Check sheet for the modelled part. Datum: model origin and axes. Units: mm. A direction names the side the tool comes from. Coordinates: 2 decimals unless noted, no trailing zeros. Loops run counter-clockwise (first coordinate to the right, second up) from the corner with the lowest first, then second, coordinate; pieces in that order, holes last. Notation, with made-up numbers: M 7.5,58.5 L 16.5,58.5 A18 ccw 16.5,65.5 Z; hole C 33.5,24 d7. An arc over 180 degrees is marked long. Return JSON: item names as keys, results as strings.
from build123d import *

# Parameters (mm, degrees)
BASE_FLANGE1_DEPTH   = 10
EDGE_FLANGE1_START   = -322.556390977
EDGE_FLANGE1_DEPTH   = 500
EDGE_FLANGE1_2_DEPTH = 500
CUT_EXTRUDE1_DEPTH   = 10


# Read off the part's stored shape, not the designer's step: Edge-Flange1
# Sheet-metal steps are written as plain solids
with BuildPart() as part:
    # Sketch1 → Base-Flange1 (new body)
    with BuildSketch(Plane.XY):
        Polygon((-322.556390977, 364.661654135), (-202.556390977, 364.661654135), (177.443609023, -45.338345865), (177.443609023, -115.338345865), (-322.556390977, -115.338345865), align=None)
    extrude(amount=-BASE_FLANGE1_DEPTH)

    # Edge-Flange1 outline → Edge-Flange1 (cut)
    with BuildSketch(Plane.YZ.offset(EDGE_FLANGE1_START)):
        with BuildLine():
            Line((-115.338345865, -10), (-111.278966663, -4.804231558))
            ThreePointArc((-111.278966663, -4.804231558), (-106.908471578, -1.265074421), (-101.428832243, 0))
            Line((-101.428832243, 0), (-115.338345865, 0))
            Line((-115.338345865, 0), (-115.338345865, -10))
        make_face()
    extrude(amount=EDGE_FLANGE1_DEPTH, mode=Mode.SUBTRACT)

    # Edge-Flange1 2 outline → Edge-Flange1 2 (add)
    with BuildSketch(Plane.YZ.offset(EDGE_FLANGE1_START)):
        with BuildLine():
            Line((-101.428832243, -10), (-115.338345865, -10))
            Line((-115.338345865, -10), (-403.042997756, -378.245161731))
            Line((-403.042997756, -378.245161731), (-395.16289022, -384.401776484))
            Line((-395.16289022, -384.401776484), (-103.398859127, -10.960846312))
            ThreePointArc((-103.398859127, -10.960846312), (-102.52476011, -10.253014884), (-101.428832243, -10))
        make_face()
    extrude(amount=EDGE_FLANGE1_2_DEPTH)

    # Sketch9 → Cut-Extrude1 (cut)
    with BuildSketch(Plane(origin=(0, -66.769129934, 52.165761512), x_dir=(1, 0, 0), z_dir=(0, -0.788010753606719, 0.6156614753256621))):
        Polygon((-202.556390977, -546.199301562), (177.443609023, -136.199301562), (177.443609023, -546.199301562), align=None)
    extrude(amount=-CUT_EXTRUDE1_DEPTH, mode=Mode.SUBTRACT)


solid = part.part
1) Go/stop test with flat-tipped pins: pin 1 Ø5 at (x, z) = (-237, -102.5) entering from +Y; pin 2 Ø12 at (x, z) = (49, -156) entering from +Y; pin 3 Ø2 at (x, y) = (-125.5, -309) entering from -Z. Record where each tip stops, or that it passes through.
Answers:
{"pin 1": "y = -172.96", "pin 2": "y = -212.03", "pin 3": "z = -275.4"}
2) Section check B-B on y = -57. Record the cut outline in (x, z), then the cut area to 3 significant figures.
Answers:
{"outline": "M -322.56,-10 L 177.44,-10 L 177.44,0 L -322.56,0 Z", "area": "5,000 mm²"}
3) Section check D-D on x = -175. Record the cut outline in (y, z), then the cut area to 3 significant figures.
Answers:
{"outline": "M -384.74,-354.82 L -376.86,-360.97 L -103.4,-10.96 A2.5 cw -101.43,-10 L 334.93,-10 L 334.93,0 L -101.43,0 A12.5 ccw -111.28,-4.8 Z", "area": "8,870 mm²"}
4) Section check A-A on x = -97. Record the cut outline in (y, z), then the cut area to 3 significant figures.
Answers:
{"outline": "M -332.93,-288.5 L -325.05,-294.66 L -103.4,-10.96 A2.5 cw -101.43,-10 L 250.77,-10 L 250.77,0 L -101.43,0 A12.5 ccw -111.28,-4.8 Z", "area": "7,190 mm²"}
5) Scan lines: line 1 along Z through (x, y) = (-241, -95.5); line 2 along Y through (x, z) = (-290, -238); line 3 along Y through (x, z) = (-4, -157.5). Record each from-to range of solid material in increasing order. Write a range as [from, to].
Answers:
{"line 1": "[-10, 0]", "line 2": "[-293.47, -280.78]", "line 3": "[-230.58, -217.89]"}
6) Set-up check for faces 1 (the face through (-125, 83, -10)), 2 (the face through (-15.216, -274.714, -222)): record each of +Z, -Z, +X, -X, +Y, -Y from which the full face is reachable in a straight line by a thin tool's end or side.
Answers:
{"face 1": "-Z, +X, -X, +Y", "face 2": "-Z, +X, -Y"}
7) Section check C-C on z = -296.5. Record the cut outline in (x, y).
Answers:
{"outline": "M -322.56,-339.18 L -106.41,-339.18 L -99.17,-326.49 L -322.56,-326.49 Z"}
